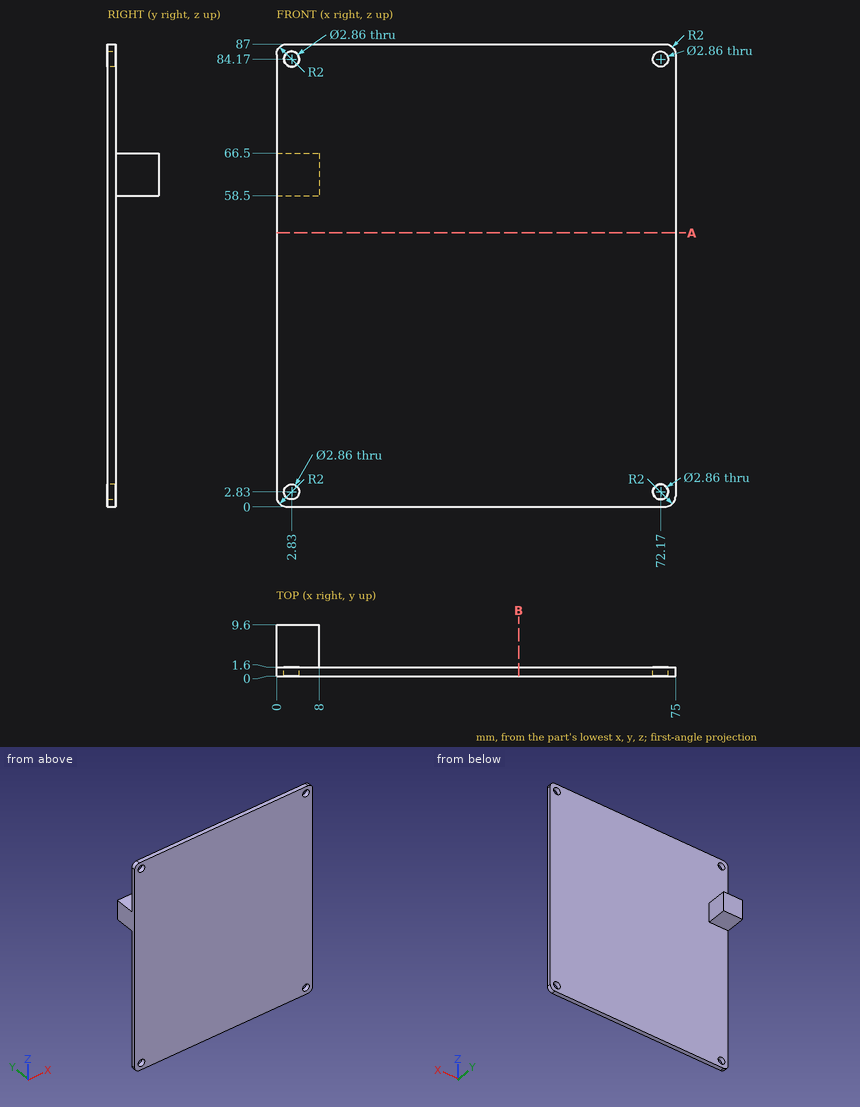
Check sheet for the drawn part. Datum: minimum x, y, z corner. Units: mm. Round coordinates to 2 decimals unless told otherwise and drop trailing zeros. Order: outer loops, then holes, each group sorted by start corner. A loop starts at its lowest first (then second) coordinate and runs counter-clockwise, first axis right, second up.
(1) Go/stop test with flat-tipped pins: P1, Ø3.5, axis at x = 72.17, z = 84.17, coming from the +Y side; P2, Ø3, axis at x = 44, z = 75, coming from the -Y side; P3, Ø2.5, axis at x = 3.5, y = 7, coming from the +Z side. Record where each tip stops, or that it passes through.
(2) Scan lines: probe 1 along X at (y, z) = (0.8, 2.83); probe 2 along Z at (x, y) = (72.17, 1.2); probe 3 along Y at (x, z) = (46, 69.5). Record each from-to range of solid material in increasing order.
(3) Cross-section at A-A, the plane z = 51.5. Enter the section's corners in (x, y).
(4) Cross-section at B-B, the plane x = 45.5. Enter the section's corners in (y, z), and give its area (3 significant figures).
Check sheet entries:
1. P1: stops at y = 1.6
1. P2: stops at y = 0
1. P3: stops at z = 66.5
2. probe 1: x = 0 to 1.4, 4.26 to 70.74, 73.6 to 75
2. probe 2: z = 0 to 1.4, 4.26 to 82.74, 85.6 to 87
2. probe 3: y = 0 to 1.6
3. outline: (0, 0) - (75, 0) - (75, 1.6) - (0, 1.6) - close
4. outline: (0, 0) - (1.6, 0) - (1.6, 87) - (0, 87) - close
4. area: 139 mm2
